The figure shows three views and two pictorial views of one solid part (mm, origin at its lowest corner). Answer the questions. A direction names the side the tool comes from. Coordinates: 2 decimals unless noted, no trailing zeros. Order: outer loops, then holes, each group sorted by start corner. A loop starts at its lowest first (then second) coordinate and runs counter-clockwise, first axis right, second up.
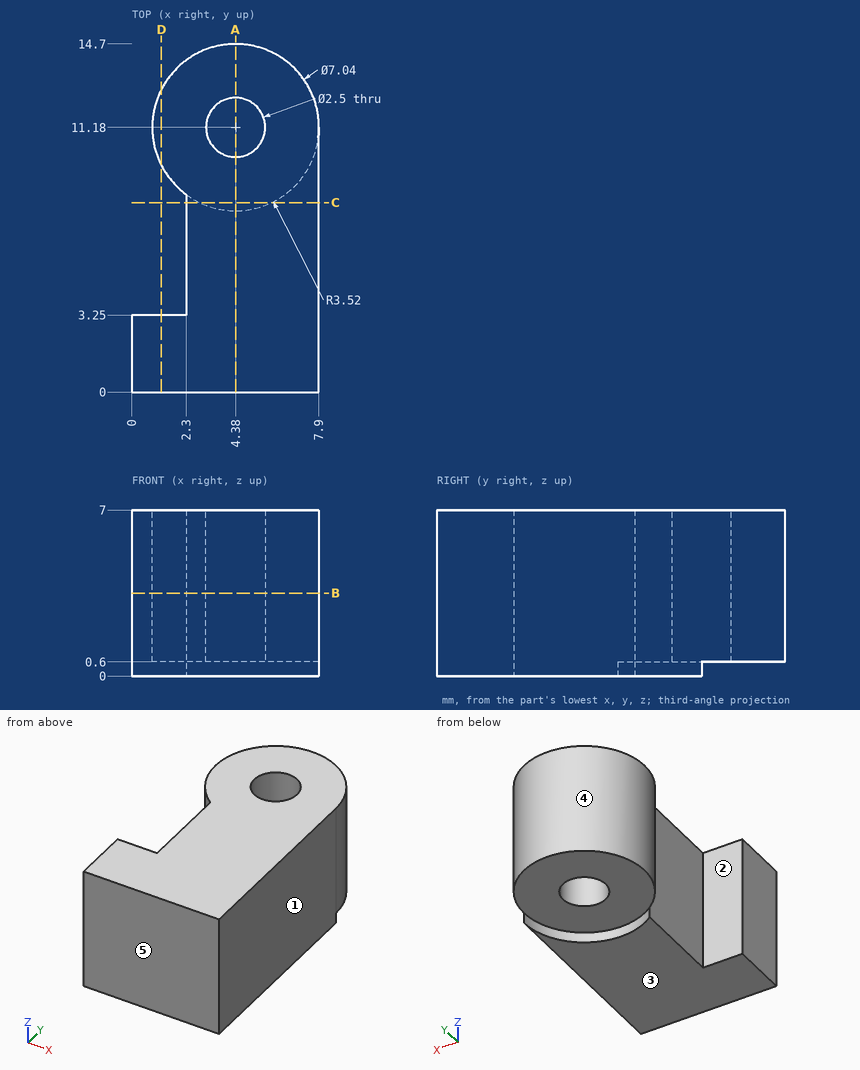
Q1. The part is cut by section C-C, the plane y = 8. Determine the outline of the cut face in (x, z), then the cut area to 3 significant figures.
Q2. Which of the six approach directions +Z, -Z, +X, -X, +Y, -Y give full straight-line access (tool end or side, diameter ignored) to the marked faces 1 and 2?
Q3. Determine the mould class of the marked faces 3, 4 and 5 for opening direction Y: +Y half, -Y half, draft (parallel to the pull), parting line (faces both ways), or undercut.
Q4. The part is cut by section A-A, the plane x = 4.38. Determine the outline of the cut face in (y, z), then the cut area to 3 significant figures.
Q5. Straight lines are drawn through the part: L1, parallel to Y at x = 4.38, z = 5.5; L2, parallel to Z at x = 1.75, y = 11.5; L3, parallel to Y at x = 4.75, z = 2.25. For each, find the intervals that lie inside material, in ascending order.
Q6. The part is cut by section D-D, the plane x = 1.25. Determine the outline of the cut face in (y, z).
Q7. Each of these flat-tipped pins is pushed along its axis until it touches: P1, Ø3.5, axis at x = 4, y = 11, coming from the -Z side; P2, Ø2.5, axis at x = 1.5, z = 5, coming from the +Y side; P3, Ø2.5, axis at y = 6.5, z = 4.5, coming from the -X side. Where does it stop, or does it pass through?
Q8. The part is cut by section B-B, the plane z = 3.5. Determine the outline of the cut face in (x, y).
Computed values:
1. outline: (2.3, 0) - (2.87, 0) - (2.87, 0.6) - (5.89, 0.6) - (5.89, 0) - (7.9, 0) - (7.9, 7) - (2.3, 7) - close
1. area: 37.4 mm2
2. face 1: +Z, -Z, +X, +Y, -Y
2. face 2: +Z, -Z, -X
3. face 3: draft
3. face 4: undercut
3. face 5: -Y half
4. outline: (0, 0) - (7.66, 0) - (7.66, 0.6) - (9.93, 0.6) - (9.93, 7) - (0, 7) - close; (12.43, 0.6) - (14.7, 0.6) - (14.7, 7) - (12.43, 7) - close
4. area: 82.7 mm2
5. L1: y = 0 to 9.93, 12.43 to 14.7
5. L2: z = 0.6 to 7
5. L3: y = 0 to 9.99, 12.37 to 14.68
6. outline: (0, 0) - (3.25, 0) - (3.25, 7) - (0, 7) - close; (9.57, 0.6) - (12.79, 0.6) - (12.79, 7) - (9.57, 7) - close
7. P1: stops at z = 0.6
7. P2: stops at y = 14.3
7. P3: stops at x = 2.3
8. outline: (0, 0) - (7.9, 0) - (7.9, 11.18) arc R3.52 ccw (long way) to (2.3, 8.34) - (2.3, 3.25) - (0, 3.25) - close; hole circle Ø2.5 at (4.38, 11.18)
